Read the model definition and answer for the solid it produces. Units are mm, in the model's axes. Face numbers are marked on the shaded views. A direction names the side the tool comes from. Give positions to 0.01 mm unless a question says otherwise; leave off trailing zeros. Write each loop counter-clockwise with the first axis right and the second up, starting at its lowest first coordinate (ties: lowest second). Pieces come first, ordered by that corner, then holes.
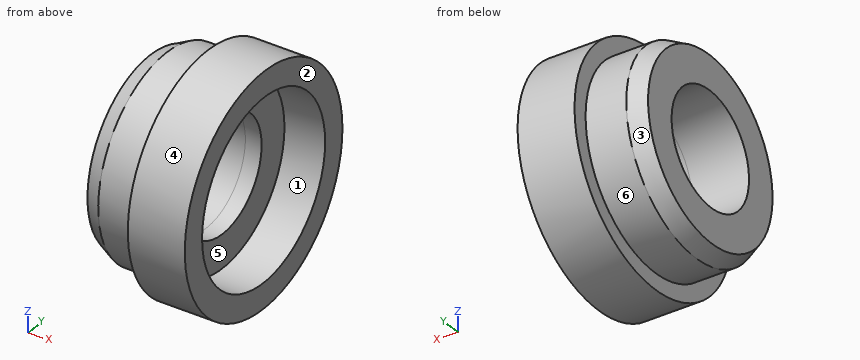
Autodesk Inventor part; units mm, degrees
ref_plane "YZ Plane" through (0, 0, 0) normal (1, 0, 0) x (0, 1, 0)
ref_plane "XZ Plane" through (0, 0, 0) normal (0, 1, 0) x (-1, 0, 0)
ref_plane "XY Plane" through (0, 0, 0) normal (0, 0, 1) x (1, 0, 0)
sketch "Sketch1" plane through (0, 0, 0) normal (1, 0, 0) x (0, 1, 0)
  circle A0 centre (0, 0) radius 11.125
  circle A1 centre (0, 0) radius 14.25
  dimension "d0" = 22.25
  dimension "d1" = 28.5
extrude "Extrusion1" add sketch "Sketch1" against normal blind 7
sketch "Sketch2" plane through (-7, 0, 0) normal (-1, 0, 0) x (0, 0, 1)
  circle A0 centre (0, 0) radius 14.25
  circle A1 centre (0, 0) radius 11.125
  circle A2 centre (0, 0) radius 12.25
  circle A3 centre (0, 0) radius 14.25
  circle A4 centre (0, 0) radius 7
  dimension "d4" = 24.5
  dimension "d5" = 14
extrude "Extrusion2" add sketch "Sketch2" along normal blind 7 contours A1 | A2
sketch "Sketch3" plane through (-7, 0, 0) normal (1, 0, 0) x (0, 0, -1)
  circle A0 centre (0, 0) radius 7
  circle A1 centre (0, 0) radius 11.125
extrude "Extrusion3" add sketch "Sketch3" along normal blind 2
chamfer "Chamfer1" distance 1 distance2 2 1 edges at (-14, 0, -12.25) measured on face at (-14, -0.9772, 10.3813)
properties part number "am3298_bearing_adapter"
Item 1: Section D-D (x = -10.75) is taken. Write down the section's boundary in (y, z).
Result set:
outline: circle Ø24.5 at (0, 0); hole circle Ø14 at (0, 0)
Item 2: Section C-C (x = -3) is taken. Write down the section's boundary in (y, z) (3 decimals).
Result set:
outline: circle Ø28.5 at (0, 0); hole circle Ø22.25 at (0, 0)
Item 3: Determine the mould class of the marked faces 1, 2 and 3 for opening direction Y: pulls with the +Y half, pulls with the -Y half, needs draft (parallel to the pull), parting line crosses it, or undercut.
Result set:
face 1: undercut
face 2: needs draft
face 3: parting line crosses it
Item 4: Which of the six approach directions +Z, -Z, +X, -X, +Y, -Y give full straight-line access (tool end or side, diameter ignored) to the marked faces 4, 5 and 6?
Result set:
face 4: +X, -X
face 5: +X
face 6: -X
Item 5: Find the intervals of material crossed by line 1 along Z through (x, y) = (-6.15, 0); line 2 along X through (y, z) = (8, -2.5); line 3 along X through (y, z) = (-7.5, -10.25), in increasing order.
Result set:
line 1: z = -14.25 to -7, 7 to 14.25
line 2: x = -14 to -5
line 3: x = -7 to 0
Item 6: Each of these flat-tipped pins is pushed along its axis until it touches: pin 1 Ø6 at (x, y) = (-11.5, 10) entering from -Z; pin 2 Ø4 at (x, y) = (-7.5, -9) entering from -Z; pin 3 Ø3 at (x, z) = (-6, 2.5) entering from -Y; pin 4 Ø12.5 at (y, z) = (0, 0) entering from -X. Where does it stop, or does it pass through?
Result set:
pin 1: stops at z = -10.05
pin 2: stops at z = -12.38
pin 3: stops at y = -14.21
pin 4: passes through
Item 7: Section A-A (y = 0) is taken. Write down the section's boundary in (x, z) (3 decimals).
Result set:
outline: (-14, -11.25) - (-12, -12.25) - (-7, -12.25) - (-7, -14.25) - (0, -14.25) - (0, -11.125) - (-5, -11.125) - (-5, -7) - (-14, -7) - close; (-14, 7) - (-5, 7) - (-5, 11.125) - (0, 11.125) - (0, 14.25) - (-7, 14.25) - (-7, 12.25) - (-12, 12.25) - (-14, 11.25) - close
